Source: CAD feature listing. Evaluate the final solid. Frame: model axes, mm. A direction names the side the tool comes from. Coordinates: 2 decimals unless noted, no trailing zeros. Write each loop counter-clockwise with the first axis right and the second up, starting at its lowest first coordinate (ties: lowest second). Pieces come first, ordered by that corner, then holes. Notation, with made-up numbers: (15, -22.5) -> (48, -22.5) arc R13 cw to (48, -0.5) -> close; hole circle Ø10 at (-17.5, 5.25). An arc over 180 degrees is marked (long way). One line per item, written item: value. Start each with the question number.
1. Line query: line 1 (Z direction, x = 4, y = -15); line 2 (Y direction, x = -3, z = 8.5); line 3 (Y direction, x = 2, z = 5). Output: solid intervals per line, ascending.
2. Section query C-C, the plane z = 5.5. Output: boundary loops of the cut face in (x, y).
3. Section query A-A, the plane y = 0. Output: boundary loops of the cut face in (x, z), and give its area (3 significant figures).
4. Section query B-B, the plane x = 0. Output: boundary loops of the cut face in (y, z), and give its area (3 significant figures).
5. Section query D-D, the plane x = 4.5. Output: boundary loops of the cut face in (y, z).
6. Mould query, pull axis X, two halves, no side actions, for faces 3 (the flat face through (20, 0, 5)), 4 (the cylindrical face through (15.975, -14.488, 5.078)), 5 (the cylindrical face through (-16.182, -13.314, 5.078)), 6 (the flat face through (9, 0, 0)). Classes: released by +X, released by -X, zero draft, split by the parting line, or undercut.
7. Access query for faces 1 (the flat face through (-9, 11, 10.3)), 2 (the cylindrical face through (16.06, 14.26, 5.08)). Directions: +Z, -Z, +X, -X, +Y, -Y. A direction counts if a zero-diameter tool reaches every point of the face in a straight line with its end or side. Return the directions, or none.
8. First-contact query: P1, Ø5, axis at x = -13.44, y = -13.44, coming from the -Z side; P2, Ø9, axis at x = 0, y = 19, coming from the +Z side; P3, Ø10, axis at y = -13, z = 30, coming from the +X side; P4, Ø8, axis at y = 1.5, z = 19, coming from the +X side. Flat tips, straight axial feed; report the tip coordinate or a pass-through.
from build123d import *

# Parameters (mm, degrees)
F0_R     = 2.75
F0_R_2   = 14
F0_R_3   = 8
F1_DEPTH = 10.3
F2_DEPTH = 42.3


with BuildPart() as f1:
    # F0 (on Top) → F1 (new body)
    with BuildSketch(Plane.XY):
        with BuildLine():
            Line((-20, 13.266499), (-20, -13.266499))
            ThreePointArc((-20, -13.266499), (0, -24), (20, -13.266499))
            Line((20, -13.266499), (20, 13.266499))
            ThreePointArc((20, 13.266499), (0, 24), (-20, 13.266499))
        make_face()
        with Locations((-13.435029, -13.435029)):
            Circle(F0_R, mode=Mode.SUBTRACT)
        with Locations((0, -19)):
            Circle(F0_R, mode=Mode.SUBTRACT)
        with Locations((13.435029, -13.435029)):
            Circle(F0_R, mode=Mode.SUBTRACT)
        with Locations((-13.435029, 13.435029)):
            Circle(F0_R, mode=Mode.SUBTRACT)
        Circle(F0_R_2, mode=Mode.SUBTRACT)
        with Locations((0, 19)):
            Circle(F0_R, mode=Mode.SUBTRACT)
        with Locations((13.435029, 13.435029)):
            Circle(F0_R, mode=Mode.SUBTRACT)
        Circle(F0_R_2)
        Circle(F0_R_3, mode=Mode.SUBTRACT)
    extrude(amount=F1_DEPTH)

    # F0 (on Top) → F2 (join)
    with BuildSketch(Plane.XY):
        Circle(F0_R_2)
        Circle(F0_R_3, mode=Mode.SUBTRACT)
    extrude(amount=F2_DEPTH)


solid = f1.part
Computed values:
1. line 1: z = 0 to 10.3
1. line 2: y = -23.81 to -7.42, 7.42 to 23.81
1. line 3: y = -23.92 to -20.89, -17.11 to -7.75, 7.75 to 17.11, 20.89 to 23.92
2. outline: (-20, -13.27) arc R24 ccw to (20, -13.27) -> (20, 13.27) arc R24 ccw to (-20, 13.27) -> close; hole circle Ø5.5 at (-13.44, -13.44); hole circle Ø5.5 at (-13.44, 13.44); hole circle Ø16 at (0, 0); hole circle Ø5.5 at (0, -19); hole circle Ø5.5 at (0, 19); hole circle Ø5.5 at (13.44, -13.44); hole circle Ø5.5 at (13.44, 13.44)
3. outline: (-20, 0) -> (-8, 0) -> (-8, 42.3) -> (-14, 42.3) -> (-14, 10.3) -> (-20, 10.3) -> close; (8, 0) -> (20, 0) -> (20, 10.3) -> (14, 10.3) -> (14, 42.3) -> (8, 42.3) -> close
3. area: 631 mm²
4. outline: (-24, 0) -> (-21.75, 0) -> (-21.75, 10.3) -> (-24, 10.3) -> close; (-16.25, 0) -> (-8, 0) -> (-8, 42.3) -> (-14, 42.3) -> (-14, 10.3) -> (-16.25, 10.3) -> close; (8, 0) -> (16.25, 0) -> (16.25, 10.3) -> (14, 10.3) -> (14, 42.3) -> (8, 42.3) -> close; (21.75, 0) -> (24, 0) -> (24, 10.3) -> (21.75, 10.3) -> close
4. area: 600 mm²
5. outline: (-23.57, 0) -> (-6.61, 0) -> (-6.61, 42.3) -> (-13.26, 42.3) -> (-13.26, 10.3) -> (-23.57, 10.3) -> close; (6.61, 0) -> (23.57, 0) -> (23.57, 10.3) -> (13.26, 10.3) -> (13.26, 42.3) -> (6.61, 42.3) -> close
6. face 3: released by +X
6. face 4: undercut
6. face 5: undercut
6. face 6: zero draft
7. face 1: +Z
7. face 2: +Z, -Z
8. P1: passes through
8. P2: stops at z = 10.3
8. P3: stops at x = 11.49
8. P4: stops at x = 14
